Here's how the part is built. I have some questions about the finished solid (model axes, mm). A direction names the side the tool comes from. Coordinates: 2 decimals unless noted, no trailing zeros. Write each loop counter-clockwise with the first axis right and the second up, starting at its lowest first coordinate (ties: lowest second). Pieces come first, ordered by that corner, then holes. Notation, with made-up numbers: M -30,-9.75 L -22,-9.75 A31 ccw -22,22.25 Z; hole C 88.5,-39.75 d3. An arc over 180 degrees is marked long. Use a Markdown table: item, result.
```python
from build123d import *

# Parameters (mm, degrees)
SKIZZE1_W                       = 100
SKIZZE1_H                       = 5
SKIZZE1_W_2                     = 300
SKIZZE1_H_2                     = 140
AUFSATZ_LINEAR_AUSTRAGEN1_DEPTH = 5
SCHNITT_LINEAR_AUSTRAGEN1_DEPTH = 168.779617356
VERRUNDUNG1_R                   = 3
SKIZZE3_W                       = 30
SKIZZE3_H                       = 75
SKIZZE3_W_2                     = 10
SKIZZE3_H_2                     = 120
SCHNITT_LINEAR_AUSTRAGEN2_DEPTH = 168.779617356


with BuildPart() as part:
    # Skizze1 → Aufsatz-Linear austragen1 (new body)
    with BuildSketch(Plane.XY):
        with Locations((0, -72.5)):
            Rectangle(SKIZZE1_W, SKIZZE1_H)
        Rectangle(SKIZZE1_W_2, SKIZZE1_H_2)
    extrude(amount=AUFSATZ_LINEAR_AUSTRAGEN1_DEPTH)

    # Skizze2 → Schnitt-Linear austragen1 (cut, through all)
    with BuildSketch(Plane.XY.offset(5)):
        Polygon((-135, 70), (115, 70), (115, 50), (70, 50), (70, 30), (65, 30), (65, 50), (20, 50), (20, 30), (15, 30), (15, 50), (-30, 50), (-30, 30), (-35, 30), (-35, 50), (-80, 50), (-80, 30), (-85, 30), (-85, 50), (-130, 50), (-130, 30), (-135, 30), (-135, 50), align=None)
    extrude(amount=-SCHNITT_LINEAR_AUSTRAGEN1_DEPTH, mode=Mode.SUBTRACT)

    # Verrundung1
    verrundung1_edges = [part.edges().sort_by_distance(p)[0] for p in [
        (70, 50, 2.5),
        (65, 50, 2.5),
        (20, 50, 2.5),
        (15, 50, 2.5),
        (-30, 50, 2.5),
        (-35, 50, 2.5),
        (-80, 50, 2.5),
        (-85, 50, 2.5),
        (-130, 50, 2.5),
    ]]
    fillet(verrundung1_edges, radius=VERRUNDUNG1_R)

    # Skizze3 → Schnitt-Linear austragen2 (cut, through all)
    with BuildSketch(Plane.XY.offset(5)):
        with Locations((-107.5, -12.5)):
            Rectangle(SKIZZE3_W, SKIZZE3_H)
        with Locations((-57.5, -12.5)):
            Rectangle(SKIZZE3_W, SKIZZE3_H)
        with Locations((-7.5, -12.5)):
            Rectangle(SKIZZE3_W, SKIZZE3_H)
        with Locations((42.5, -12.5)):
            Rectangle(SKIZZE3_W, SKIZZE3_H)
        with Locations((92.5, -12.5)):
            Rectangle(SKIZZE3_W, SKIZZE3_H)
        with Locations((130, 0)):
            Rectangle(SKIZZE3_W_2, SKIZZE3_H_2)
    extrude(amount=-SCHNITT_LINEAR_AUSTRAGEN2_DEPTH, mode=Mode.SUBTRACT)


solid = part.part
```
1. Suppose I cut it at C-C on y = 36. Write out the boundary of the cut face in (x, z).
Answers follow:
| item | result |
|---|---|
| outline | M -150,0 L -135,0 L -135,5 L -150,5 Z; M -130,0 L -85,0 L -85,5 L -130,5 Z; M -80,0 L -35,0 L -35,5 L -80,5 Z; M -30,0 L 15,0 L 15,5 L -30,5 Z; M 20,0 L 65,0 L 65,5 L 20,5 Z; M 70,0 L 125,0 L 125,5 L 70,5 Z; M 135,0 L 150,0 L 150,5 L 135,5 Z |
2. Suppose I cut it at B-B on x = -111. Write out the boundary of the cut face in (y, z), and give its area (3 significant figures).
Answers follow:
| item | result |
|---|---|
| outline | M -70,0 L -50,0 L -50,5 L -70,5 Z; M 25,0 L 50,0 L 50,5 L 25,5 Z |
| area | 225 mm2 |
3. Will these pins go through, and if not, where does the flat tip stop? pin 1 Ø2.5 at (x, z) = (-83, 2.5) entering from -Y; pin 2 Ø2.5 at (x, z) = (-51, 3.5) entering from +Y.
Answers follow:
| item | result |
|---|---|
| pin 1 | stops at y = -70 |
| pin 2 | stops at y = 50 |
4. Which directions (+Z, -Z, +X, -X, +Y, -Y) give clear straight access to the entire face, cutting with the end or side of a thin tool? Please do faces 1 (the face through (-130, 39, 3)), 2 (the face through (150, -1, 2)), 3 (the face through (-50, -73, 2)), 4 (the face through (130, 60, 3)), 5 (the face through (99, -70, 2)).
Answers follow:
| item | result |
|---|---|
| face 1 | +Z, -Z, +Y |
| face 2 | +Z, -Z, +X, +Y, -Y |
| face 3 | +Z, -Z, -X, -Y |
| face 4 | +Z, -Z |
| face 5 | +Z, -Z, +X, -Y |
5. We'd pull the mould along X, two halves only. Please class faces 6 (the face through (-80, 39, 3)), 7 (the face through (132, 70, 2)), 8 (the face through (50, -73, 2)), 9 (the face through (-7, 50, 3)): +X half, -X half, draft (parallel to the pull), parting line (faces both ways), or undercut.
Answers follow:
| item | result |
|---|---|
| face 6 | undercut |
| face 7 | draft |
| face 8 | +X half |
| face 9 | undercut |
6. Suppose I cut it at D-D on z = 2.05. State how many separate pieces and enclosed holes the cut face has, and give its area (3 significant figures).
Answers follow:
| item | result |
|---|---|
| separate pieces | 1 |
| enclosed holes | 6 |
| area | 24,500 mm2 |
7. I need wall thicknesses on probe 1 along X at (y, z) = (56, 3.2); probe 2 along X at (y, z) = (-53.5, 4.55); probe 3 along Y at (x, z) = (-51.5, 0.3). Which ranges of each line are inside material? Lowest first, please.
Answers follow:
| item | result |
|---|---|
| probe 1 | x = -150 to -135, 115 to 125, 135 to 150 |
| probe 2 | x = -150 to 125, 135 to 150 |
| probe 3 | y = -70 to -50, 25 to 50 |
8. Suppose I cut it at A-A on y = 53.5. Write out the boundary of the cut face in (x, z), and give its area (3 significant figures).
Answers follow:
| item | result |
|---|---|
| outline | M -150,0 L -135,0 L -135,5 L -150,5 Z; M 115,0 L 125,0 L 125,5 L 115,5 Z; M 135,0 L 150,0 L 150,5 L 135,5 Z |
| area | 200 mm2 |
